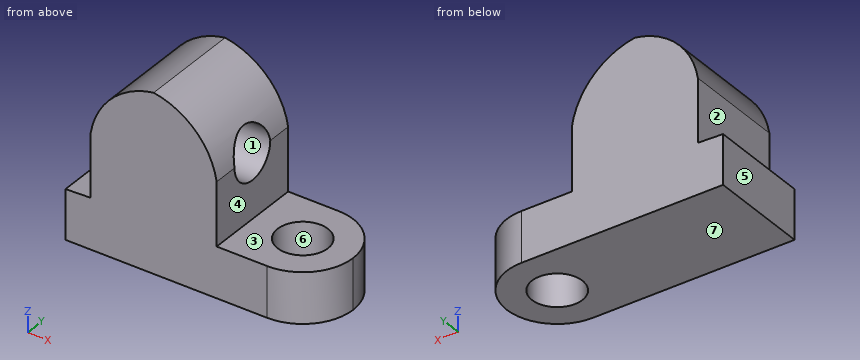
```python
from build123d import *

# Parameters (mm, degrees)
F1_DEPTH = 25.4
F3_DEPTH = 25.4
F4_R     = 6.35
F5_DEPTH = 25.4
F7_DEPTH = 25.4
F9_DEPTH = 25.4


# Not quite as in the source:
# - ends of sketch curves that miss each other by under 0.0002 mm in the source are joined


with BuildPart() as f1:
    # F0 (on Front) → F1 (new body)
    with BuildSketch(Plane.XZ):
        Polygon((-67.7254482706, 28.6358930171), (-67.7254482706, 16.1884303746), (-4.2254482706, 16.1884303746), (-4.2254482706, 28.8884303746), (-29.6254482706, 28.8884303746), (-29.6254482706, 60.6384303746), (-61.3754482706, 60.6384303746), (-61.3754482706, 28.8884303746), align=None)
    extrude(amount=F1_DEPTH)

    # F2 (on face) → F3 (cut)
    with BuildSketch(Plane.XY.offset(28.8884303746)):
        with BuildLine():
            ThreePointArc((-16.9254482706, 0), (-7.9451915343, -3.7197435424), (-4.2254473189, -12.7))
            Line((-4.2254473189, -12.7), (-4.2254482706, 0))
            Line((-4.2254482706, 0), (-16.9254482706, 0))
        make_face()
        with BuildLine():
            ThreePointArc((-4.2254473189, -12.7), (-7.9451908613, -21.6802557846), (-16.9254463672, -25.4))
            Line((-16.9254463672, -25.4), (-4.2254482706, -25.4))
            Line((-4.2254482706, -25.4), (-4.2254473189, -12.7))
        make_face()
    extrude(amount=-F3_DEPTH, mode=Mode.SUBTRACT)

    # F4 (on face) → F5 (cut)
    with BuildSketch(Plane.XY.offset(28.8884303746)):
        with Locations((-16.9254473189, -12.7)):
            Circle(F4_R)
    extrude(amount=-F5_DEPTH, mode=Mode.SUBTRACT)

    # F6 (on face) → F7 (cut)
    with BuildSketch(Plane.XZ.offset(25.4)):
        with BuildLine():
            ThreePointArc((-45.5004482706, 60.6384303746), (-34.9759157672, 55.287962878), (-29.6254482706, 44.7634303746))
            Line((-29.6254482706, 44.7634303746), (-29.6254482706, 60.6384303746))
            Line((-29.6254482706, 60.6384303746), (-45.5004482706, 60.6384303746))
        make_face()
        with BuildLine():
            ThreePointArc((-61.3754482706, 44.7634303746), (-56.0249807741, 55.287962878), (-45.5004482706, 60.6384303746))
            Line((-45.5004482706, 60.6384303746), (-61.3754482706, 60.6384303746))
            Line((-61.3754482706, 60.6384303746), (-61.3754482706, 44.7634303746))
        make_face()
    extrude(amount=-F7_DEPTH, mode=Mode.SUBTRACT)

    # F8 (on face) → F9 (cut)
    with BuildSketch(Plane.YZ.offset(-29.6254482706)):
        with BuildLine():
            ThreePointArc((-19.05, 44.7634303746), (-12.7, 38.4134303746), (-6.35, 44.7634303746))
            Line((-6.35, 44.7634303746), (-19.05, 44.7634303746))
        make_face()
        with BuildLine():
            Line((-19.05, 44.7634303746), (-6.35, 44.7634303746))
            ThreePointArc((-6.35, 44.7634303746), (-12.7, 51.1134303746), (-19.05, 44.7634303746))
        make_face()
    extrude(amount=-F9_DEPTH, mode=Mode.SUBTRACT)


solid = f1.part
```
Part model, mm, in its own coordinate system. Face numbers are marked on the shaded views. A direction names the side the tool comes from. Round coordinates to 2 decimals unless told otherwise and drop trailing zeros. Loops run counter-clockwise (first coordinate to the right, second up) from the corner with the lowest first, then second, coordinate; pieces in that order, holes last.
Item 1: 3-axis set-ups, long thin cutter, end or side, ignore diameter. For the marked faces 1, 2 and 3: which of +Z, -Z, +X, -X, +Y, -Y reach the whole face in a straight line?
Item 2: Cut at B-B, the plane x = -40. Give the cut face in (y, z).
Item 3: Cut at C-C, the plane y = -21.25. Give the cut face in (x, z), then the cut area to 3 significant figures.
Item 4: Cut at D-D, the plane z = 37. Give the cut face in (x, y).
Item 5: Cut at A-A, the plane y = -9.5. Give the cut face in (x, z), then the cut area to 3 significant figures.
Item 6: Drop flat-ended pins along their axis: P1, Ø12.5, axis at y = -18.5, z = 37.5, coming from the +X side; P2, Ø10, axis at y = -12.7, z = 44.76, coming from the +X side; P3, Ø10, axis at y = -3, z = 45, coming from the -X side; P4, Ø12, axis at x = -22.5, z = 39.5, coming from the -Y side. Give the stop position or say it passes through.
Item 7: Mould opens along X. For the marked faces 4, 5, 6 and 7 say: +X half, -X half, draft (parallel to the pull), parting line (faces both ways), or undercut.
Item 8: Drill centre lines: line 1 (X direction, y = -8, z = 20.5); line 2 (Z direction, x = -14.5, y = -23.5); line 3 (Z direction, x = -53.5, y = -8.25). Where is each one in solid material? Low to high.
A:
1. face 1: +X
1. face 2: +Z, -X, +Y, -Y
1. face 3: +Z, +X, +Y, -Y
2. outline: (-25.4, 16.19) - (0, 16.19) - (0, 58.89) - (-25.4, 58.89) - close; hole circle Ø12.7 at (-12.7, 44.76)
3. outline: (-67.73, 16.19) - (-7.53, 16.19) - (-7.53, 28.89) - (-29.63, 28.89) - (-29.63, 44.76) arc R19.05 ccw to (-45.5, 60.64) arc R19.05 ccw to (-61.38, 44.76) - (-61.38, 28.89) - (-67.73, 28.64) - close
3. area: 1,630 mm2
4. outline: (-61.38, -25.4) - (-29.63, -25.4) - (-29.63, 0) - (-61.38, 0) - close
5. outline: (-67.73, 16.19) - (-22.41, 16.19) - (-22.41, 28.89) - (-29.63, 28.89) - (-29.63, 39.28) - (-55.03, 39.28) - (-55.03, 50.25) - (-31.36, 50.25) arc R19.05 ccw to (-45.5, 60.64) arc R19.05 ccw to (-61.38, 44.76) - (-61.38, 28.89) - (-67.73, 28.64) - close; (-11.44, 16.19) - (-4.64, 16.19) - (-4.64, 28.89) - (-11.44, 28.89) - close
5. area: 1,250 mm2
6. P1: stops at x = -29.63
6. P2: stops at x = -55.03
6. P3: stops at x = -61.38
6. P4: passes through
7. face 4: +X half
7. face 5: -X half
7. face 6: undercut
7. face 7: draft
8. line 1: x = -67.73 to -21.2, -12.66 to -5.13
8. line 2: z = 16.19 to 28.89
8. line 3: z = 16.19 to 40.23, 49.29 to 57.41
